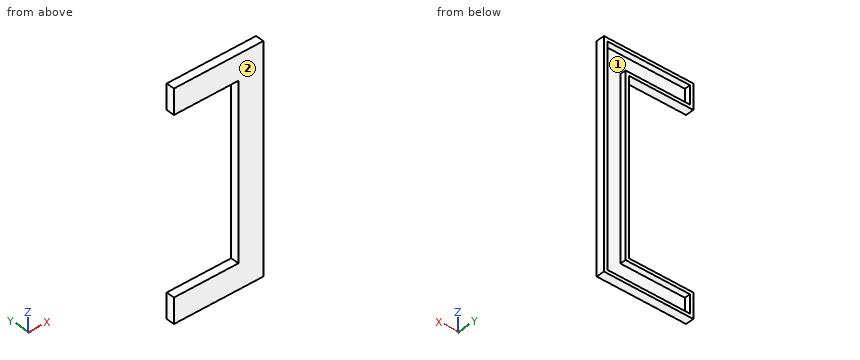
from build123d import *

# Parameters (mm, degrees)
BOSS_EXTRUDE1_DEPTH = 4
CUT_EXTRUDE1_DEPTH  = 2.8


with BuildPart() as part:
    # Sketch1 → Boss-Extrude1 (new body)
    with BuildSketch(Plane(origin=(0, 0, 0), x_dir=(1, 0, 0), z_dir=(0, 1, 0))):
        Polygon((0, 106.68), (43.06, 106.68), (43.06, 0), (0, 0), (0, 12), (31.06, 12), (31.06, 94.68), (0, 94.68), align=None)
    extrude(amount=BOSS_EXTRUDE1_DEPTH)

    # Sketch2 → Cut-Extrude1 (cut)
    with BuildSketch(Plane(origin=(0, 4, 0), x_dir=(1, 0, 0), z_dir=(0, 1, 0))):
        Polygon((1.6, 105.08), (1.6, 96.28), (32.66, 96.28), (32.66, 10.4), (1.6, 10.4), (1.6, 1.6), (41.46, 1.6), (41.46, 105.08), align=None)
    extrude(amount=-CUT_EXTRUDE1_DEPTH, mode=Mode.SUBTRACT)


solid = part.part
Could you check a few things on this model? Use its own coordinates, in mm. Face numbers are marked on the shaded views. Give positions to 0.01 mm unless a question says otherwise; leave off trailing zeros. Order: outer loops, then holes, each group sorted by start corner. A loop starts at its lowest first (then second) coordinate and runs counter-clockwise, first axis right, second up. Notation, with made-up numbers: M -1,-15.5 L 33,-15.5 A20 ccw 33,4.5 Z; hole C -18,-19 d2. An arc over 180 degrees is marked long. One line per question, with ' | ' between items.
1. If I drill on line 1 (Z direction, x = 7, y = 2.3); line 2 (Z direction, x = 10, y = 0.2); line 3 (X direction, y = 2.3, z = -89), over which ranges is the centre line in solid material (lowest first)?
Results:
line 1: -106.68 to -105.08, -96.28 to -94.68, -12 to -10.4, -1.6 to 0 | line 2: -106.68 to -94.68, -12 to 0 | line 3: 31.06 to 32.66, 41.46 to 43.06
2. I want a section at B-B (y = 2.95). List the corners of the cut face in (x, z) for me.
Results:
outline: M 0,-106.68 L 43.06,-106.68 L 43.06,0 L 0,0 L 0,-12 L 31.06,-12 L 31.06,-94.68 L 0,-94.68 Z; hole M 1.6,-105.08 L 41.46,-105.08 L 41.46,-1.6 L 1.6,-1.6 L 1.6,-10.4 L 32.66,-10.4 L 32.66,-96.28 L 1.6,-96.28 Z
3. I want a section at C-C (z = -16). List the corners of the cut face in (x, y) for me.
Results:
outline: M 31.06,0 L 43.06,0 L 43.06,4 L 41.46,4 L 41.46,1.2 L 32.66,1.2 L 32.66,4 L 31.06,4 Z
4. I want a section at A-A (x = 17.5). List the corners of the cut face in (y, z) for me.
Results:
outline: M 0,-106.68 L 4,-106.68 L 4,-105.08 L 1.2,-105.08 L 1.2,-96.28 L 4,-96.28 L 4,-94.68 L 0,-94.68 Z; M 0,-12 L 4,-12 L 4,-10.4 L 1.2,-10.4 L 1.2,-1.6 L 4,-1.6 L 4,0 L 0,0 Z
5. We'd pull the mould along X, two halves only. Please class the marked faces 1 and 2: +X half, -X half, draft (parallel to the pull), parting line (faces both ways), or undercut.
Results:
face 1: undercut | face 2: draft
6. I'm going to push flat-ended pins straight in: pin 1 (2 mm diameter, centred on y = 2, z = -39.5, fed in from -X); pin 2 (0.8 mm diameter, centred on x = 10.5, y = 2.5, fed in from +Z). Where does each tip first touch, or does it pass through?
Results:
pin 1: x = 31.06 | pin 2: z = 0
7. I want a section at D-D (x = 38.5). List the corners of the cut face in (y, z) for me, and give its area (3 significant figures).
Results:
outline: M 0,-106.68 L 4,-106.68 L 4,-105.08 L 1.2,-105.08 L 1.2,-1.6 L 4,-1.6 L 4,0 L 0,0 Z | area: 137 mm²
